```python
from build123d import *

# Parameters (mm, degrees)
VACIADO1_T            = -2.5
CORTAR_EXTRUIR5_REACH = 223.133
CROQUIS2_R            = 1.5
CROQUIS2_R_2          = 6.175
CROQUIS9_R            = 10
CORTAR_EXTRUIR9_DEPTH = 10


with BuildPart() as part:
    # Croquis1 → Revolución1 (revolve)
    with BuildSketch(Plane(origin=(0, 0, 0), x_dir=(1, 0, 0), z_dir=(0, 1, 0)), mode=Mode.PRIVATE) as revoluci_n1_sk:
        Polygon((0, -85), (0, 85), (-88, 85), (-100, -85), align=None)
    revolve(revoluci_n1_sk.sketch.rotate(Axis((0, 0, 85), (0, 0, -1)), 180), axis=Axis((0, 0, 85), (0, 0, -1)))

    # Vaciado1
    vaciado1_openings = [part.faces().sort_by_distance(p)[0] for p in [
        (0, 0, -85),
    ]]
    offset(amount=VACIADO1_T, openings=vaciado1_openings, kind=Kind.INTERSECTION)

    # Croquis2 → Cortar-Extruir5 (cut, up to next)
    with BuildSketch(Plane.XY.offset(85), mode=Mode.PRIVATE) as cortar_extruir5_sk1:
        Circle(CROQUIS2_R)
    cortar_extruir5_tool1 = extrude(cortar_extruir5_sk1.sketch, amount=-CORTAR_EXTRUIR5_REACH, mode=Mode.PRIVATE) & part.part
    # Croquis2 → Cortar-Extruir5 (cut, up to next)
    with BuildSketch(Plane.XY.offset(85), mode=Mode.PRIVATE) as cortar_extruir5_sk2:
        with Locations((-24.5, 0)):
            Circle(CROQUIS2_R_2)
    cortar_extruir5_tool2 = extrude(cortar_extruir5_sk2.sketch, amount=-CORTAR_EXTRUIR5_REACH, mode=Mode.PRIVATE) & part.part
    # Croquis2 → Cortar-Extruir5 (cut, up to next)
    with BuildSketch(Plane.XY.offset(85), mode=Mode.PRIVATE) as cortar_extruir5_sk3:
        with Locations((24.5, 0)):
            Circle(CROQUIS2_R_2)
    cortar_extruir5_tool3 = extrude(cortar_extruir5_sk3.sketch, amount=-CORTAR_EXTRUIR5_REACH, mode=Mode.PRIVATE) & part.part
    add(cortar_extruir5_tool1.solids().sort_by_distance((0, 0, 85))[0], mode=Mode.SUBTRACT)
    add(cortar_extruir5_tool2.solids().sort_by_distance((-24.5, 0, 85))[0], mode=Mode.SUBTRACT)
    add(cortar_extruir5_tool3.solids().sort_by_distance((24.5, 0, 85))[0], mode=Mode.SUBTRACT)

    # Croquis9 → Cortar-Extruir9 (cut)
    with BuildSketch(Plane.XY.offset(85)):
        with Locations((0, 68.666733176)):
            Circle(CROQUIS9_R)
        with Locations((48.55471267, 48.55471267)):
            Circle(CROQUIS9_R)
        with Locations((68.666733176, 0)):
            Circle(CROQUIS9_R)
        with Locations((48.55471267, -48.55471267)):
            Circle(CROQUIS9_R)
        with Locations((0, -68.666733176)):
            Circle(CROQUIS9_R)
        with Locations((-48.55471267, -48.55471267)):
            Circle(CROQUIS9_R)
        with Locations((-68.666733176, 0)):
            Circle(CROQUIS9_R)
        with Locations((-48.55471267, 48.55471267)):
            Circle(CROQUIS9_R)
    extrude(amount=-CORTAR_EXTRUIR9_DEPTH, mode=Mode.SUBTRACT)


solid = part.part
```
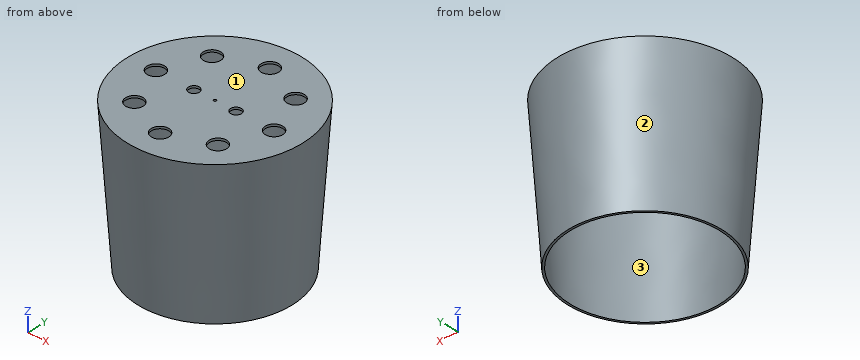
CAD build for the part. Positions are in the model's coordinates, mm. Face numbers are marked on the shaded views. Coordinates: 2 decimals unless noted, no trailing zeros. Order: outer loops, then holes, each group sorted by start corner. A loop starts at its lowest first (then second) coordinate and runs counter-clockwise, first axis right, second up. Notation, with made-up numbers: (14.5, 31) -> (66.5, 31) arc R25 ccw to (66.5, 58) -> close; hole circle Ø3 at (-21, 66.5). An arc over 180 degrees is marked (long way). Use one line per item in the form item = value. Start each with the question number.
1) Drop flat-ended pins along their axis: pin 1 (3 mm diameter, centred on x = 36.5, z = 66, fed in from -Y); pin 2 (4 mm diameter, centred on y = 57.5, z = 39, fed in from -X); pin 3 (16 mm diameter, centred on x = 24.5, y = 0, fed in from +Z); pin 4 (12 mm diameter, centred on x = 6.5, y = 64, fed in from -Z). Give the stop position or say it passes through.
2) Drill centre lines: L1, parallel to Y at x = -24.5, z = 84.45 (3 decimals); L2, parallel to Z at x = 34.5, y = -56; L3, parallel to Y at x = 69, z = 48. Where is each one in solid material? Low to high. Write a range as [from, to].
3) Band-saw the part on A-A on z = 69. Give the cut face in (x, y).
4) Band-saw the part on C-C on z = -44. Give the cut face in (x, y), then the cut area to 3 significant figures.
5) Band-saw the part on B-B on y = 53.5. State how many separate pieces and enclosed holes the cut face has, then the cut area to 3 significant figures.
6) Pull direction Y, two halves, no side cores. Call the marked faces 1, 2 and 3: +Y half, -Y half, draft (parallel to the pull), parting line (faces both ways), or undercut.
Entries:
q1.pin_1 = -92.25
q1.pin_2 = -79.26
q1.pin_3 = 85
q1.pin_4 = 82.5
q2.L1 = [-96.912, -6.175], [6.175, 96.912]
q2.L2 = [82.5, 85]
q2.L3 = [-68.73, -65.13], [65.13, 68.73]
q3.outline = circle Ø197.74 at (0, 0); hole circle Ø192.73 at (0, 0)
q4.outline = circle Ø181.79 at (0, 0); hole circle Ø176.78 at (0, 0)
q4.area = 1,410 mm2
q5.separate_pieces = 3
q5.enclosed_holes = 0
q5.area = 1,360 mm2
q6.face_1 = draft
q6.face_2 = parting line
q6.face_3 = undercut
